Geometry check sheet. Reference: the model listing, model coordinates, mm. Face numbers are marked on the shaded views. A direction names the side the tool comes from. Round coordinates to 2 decimals unless told otherwise and drop trailing zeros. Loops run counter-clockwise (first coordinate to the right, second up) from the corner with the lowest first, then second, coordinate; pieces in that order, holes last. Notation, with made-up numbers: (15, -14) - (62, -14) arc R33 cw to (62, 15) - close; hole circle Ø7 at (63.5, 18). An arc over 180 degrees is marked (long way). Answer as CSV lines item,"result". Start each with the question number.
1) Cross-section at A-A on x = 0. Record the boundary of the cut face in (y, z).
2) Cross-section at B-B on y = -2. Record the boundary of the cut face in (x, z), and give its area (3 significant figures).
3) Access from +Z, -Z, +X, -X, +Y, -Y to the whole of each face (thin tool, end or side, straight path). Record for the marked faces 1 and 2.
4) Draft check along Z on the marked faces 3, 4, 5 and 6. Enter one of: released by +Z, released by -Z, zero draft, split by the parting line, or undercut.
5) Cross-section at C-C on y = -15.25. Record the boundary of the cut face in (x, z).
6) Thickness scan on line 1 along Z through (x, y) = (0, -13.75); line 2 along Y through (x, z) = (-1, 0.25); line 3 along Y through (x, z) = (-1.25, -1.5). Record the ranges inside material, lowest first.
7) Depth check by flat-ended pin: P1, Ø3, axis at y = -6, z = -1.5, coming from the -X side; P2, Ø1.5, axis at x = 2, y = -7.5, coming from the +Z side; P3, Ø2, axis at x = -2, y = -10, coming from the +Z side; P4, Ø1, axis at x = 0.5, y = -3, coming from the +Z side. Enter the tip coordinate at first touch or a pass-through.
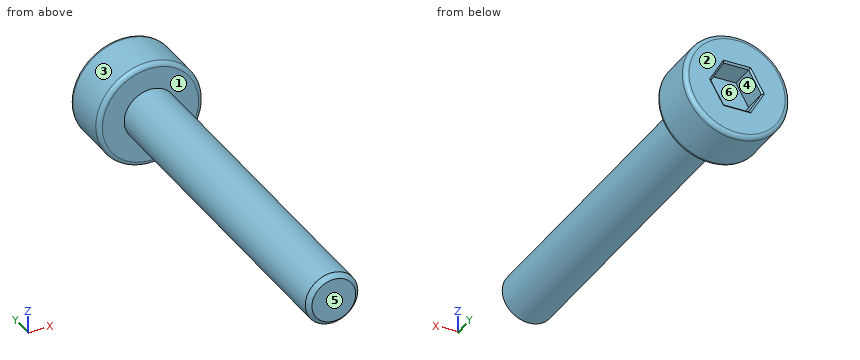
Autodesk Inventor part; units mm, degrees
ref_plane "YZ Plane" through (0, 0, 0) normal (1, 0, 0) x (0, 1, 0)
ref_plane "XZ Plane" through (0, 0, 0) normal (0, 1, 0) x (-1, 0, 0)
ref_plane "XY Plane" through (0, 0, 0) normal (0, 0, 1) x (1, 0, 0)
sketch "Sketch1" plane through (0, 0, 0) normal (0, 1, 0) x (-1, 0, 0)
  circle A0 centre (0, 0) radius 3
  dimension "d0" = 6
extrude "Extrusion1" add sketch "Sketch1" against normal blind 3
sketch "Sketch2" plane through (0, -3, 0) normal (0, -1, 0) x (1, 0, 0)
  circle A0 centre (0, 0) radius 1.5
  dimension "d3" = 3
extrude "Extrusion2" add sketch "Sketch2" along normal blind 20
sketch "Sketch3" plane through (0, 0, 0) normal (0, 1, 0) x (1, 0, 0)
  circle A0 centre (0, 0) radius 1.5 construction
  line L0 (1.4434, 0) -> (0.7217, -1.25)
  line L1 (0.7217, -1.25) -> (-0.7217, -1.25)
  line L2 (-0.7217, -1.25) -> (-1.4434, 0)
  line L3 (-1.4434, 0) -> (-0.7217, 1.25)
  line L4 (-0.7217, 1.25) -> (0.7217, 1.25)
  line L5 (0.7217, 1.25) -> (1.4434, 0)
  dimension "d8" = 2.5
extrude "Extrusion3" cut sketch "Sketch3" against normal blind 1.5
chamfer "Chamfer1" distance 0.25 angle 45 1 edges at (-1.5, -23, 0)
fillet "Fillet1" radius 0.25 2 edges at (3, 0, 0) (3, -3, 0)
chamfer "Chamfer2" distance 0.1 angle 45 6 edges at (0, 0, -1.25) (1.0825, 0, -0.625) (1.0825, 0, 0.625) (0, 0, 1.25) (-1.0825, 0, 0.625) (-1.0825, 0, -0.625)
thread "Thread2"
properties part number "M3-20" material "Steel, Carbon"
Answer block:
1,outline,"(-23, -1.25) - (-22.75, -1.5) - (-3, -1.5) - (-3, -2.75) arc R0.25 ccw to (-2.75, -3) - (-0.25, -3) arc R0.25 ccw to (0, -2.75) - (0, -1.35) - (-0.1, -1.25) - (-1.5, -1.25) - (-1.5, 1.25) - (-0.1, 1.25) - (0, 1.35) - (0, 2.75) arc R0.25 ccw to (-0.25, 3) - (-2.75, 3) arc R0.25 ccw to (-3, 2.75) - (-3, 1.5) - (-22.75, 1.5) - (-23, 1.25) - close"
2,outline,"circle Ø6 at (0, 0)"
2,area,"28.3 mm^2"
3,face 1,"-Y"
3,face 2,"+Z, -Z, +X, -X, +Y"
4,face 3,"split by the parting line"
4,face 4,"undercut"
4,face 5,"zero draft"
4,face 6,"undercut"
5,outline,"circle Ø3 at (0, 0)"
6,line 1,"z = -1.5 to 1.5"
6,line 2,"y = -23 to -1.5"
6,line 3,"y = -3 to 0"
7,P1,"stops at x = -1.5"
7,P2,"stops at z = 0.83"
7,P3,"stops at z = 1.12"
7,P4,"stops at z = 3"
